from build123d import *

# Parameters (mm, degrees)
SKETCH1_R           = 50
SKETCH1_R_2         = 11.05
SKETCH1_R_3         = 1.55
BOSS_EXTRUDE1_DEPTH = 10
BOSS_EXTRUDE2_START = -2.9
SKETCH2_R           = 11.05
SKETCH2_R_2         = 4.05
BOSS_EXTRUDE2_DEPTH = 2.9


with BuildPart() as part:
    # Sketch1 → Boss-Extrude1 (new body)
    with BuildSketch(Plane.XY):
        Circle(SKETCH1_R)
        Circle(SKETCH1_R_2, mode=Mode.SUBTRACT)
        with Locations((40, 0)):
            Circle(SKETCH1_R_3, mode=Mode.SUBTRACT)
        with Locations((33.650141313, -21.625632698)):
            Circle(SKETCH1_R_3, mode=Mode.SUBTRACT)
        with Locations((16.61660052, -36.385279814)):
            Circle(SKETCH1_R_3, mode=Mode.SUBTRACT)
        with Locations((-5.692593531, -39.592857675)):
            Circle(SKETCH1_R_3, mode=Mode.SUBTRACT)
        with Locations((-26.194429358, -30.229982974)):
            Circle(SKETCH1_R_3, mode=Mode.SUBTRACT)
        with Locations((-38.379718945, -11.269302274)):
            Circle(SKETCH1_R_3, mode=Mode.SUBTRACT)
        with Locations((-38.379718945, 11.269302274)):
            Circle(SKETCH1_R_3, mode=Mode.SUBTRACT)
        with Locations((-26.194429358, 30.229982974)):
            Circle(SKETCH1_R_3, mode=Mode.SUBTRACT)
        with Locations((-5.692593531, 39.592857675)):
            Circle(SKETCH1_R_3, mode=Mode.SUBTRACT)
        with Locations((16.61660052, 36.385279814)):
            Circle(SKETCH1_R_3, mode=Mode.SUBTRACT)
        with Locations((33.650141313, 21.625632698)):
            Circle(SKETCH1_R_3, mode=Mode.SUBTRACT)
    extrude(amount=BOSS_EXTRUDE1_DEPTH)

    # Sketch2 → Boss-Extrude2 (add)
    with BuildSketch(Plane.XY.offset(10).offset(BOSS_EXTRUDE2_START)):
        Circle(SKETCH2_R)
        Circle(SKETCH2_R_2, mode=Mode.SUBTRACT)
    extrude(amount=BOSS_EXTRUDE2_DEPTH)


solid = part.part
Here's how the part is built. I have some questions about the finished solid (model axes, mm). A direction names the side the tool comes from. Coordinates: 2 decimals unless noted, no trailing zeros. Write each loop counter-clockwise with the first axis right and the second up, starting at its lowest first coordinate (ties: lowest second). Pieces come first, ordered by that corner, then holes.
1) Thinking about a two-plate mould opening in X: for faces 3 (the face through (-12, 1, 0)), 4 (the face through (34.365, 20.251, 4.93)), 5 (the face through (-5.89, 41.13, 4.93)), 6 (the face through (47.69, 15.02, 4.93)), which applies, +X half, -X half, draft (parallel to the pull), parting line (faces both ways), or undercut?
Filled in:
face 3: draft
face 4: undercut
face 5: undercut
face 6: parting line
2) If we section it at A-A (x = 40): List the corners of the cut face in (y, z) for me, plus the area to 3 significant figures.
Filled in:
outline: (-30, 0) - (-1.55, 0) - (-1.55, 10) - (-30, 10) - close; (1.55, 0) - (30, 0) - (30, 10) - (1.55, 10) - close
area: 569 mm2
3) If we section it at D-D (x = 0): List the corners of the cut face in (y, z) for me.
Filled in:
outline: (-50, 0) - (-11.05, 0) - (-11.05, 7.1) - (-4.05, 7.1) - (-4.05, 10) - (-50, 10) - close; (4.05, 7.1) - (11.05, 7.1) - (11.05, 0) - (50, 0) - (50, 10) - (4.05, 10) - close
4) I'm going to push flat-ended pins straight in: pin 1 (4 mm diameter, centred on y = -3.5, z = 2.5, fed in from -X); pin 2 (4 mm diameter, centred on x = -23.5, z = 7.5, fed in from -Y); pin 3 (3.5 mm diameter, centred on x = 16.62, y = 36.39, fed in from -Z); pin 4 (11 mm diameter, centred on x = 2, y = 0, fed in from -Z). Where does each tip first touch, or does it pass through?
Filled in:
pin 1: stops at x = -49.98
pin 2: stops at y = -45.14
pin 3: stops at z = 0
pin 4: stops at z = 7.1
5) Which directions (+Z, -Z, +X, -X, +Y, -Y) give clear straight access to the entire face, cutting with the end or side of a thin tool? Please do faces 1 (the face through (-1, -10, 10)), 2 (the face through (0, -5, 7.1)).
Filled in:
face 1: +Z, +X, -X, +Y, -Y
face 2: -Z
6) If we section it at B-B (y = 0): List the corners of the cut face in (x, z) for me.
Filled in:
outline: (-50, 0) - (-11.05, 0) - (-11.05, 7.1) - (-4.05, 7.1) - (-4.05, 10) - (-50, 10) - close; (4.05, 7.1) - (11.05, 7.1) - (11.05, 0) - (38.45, 0) - (38.45, 10) - (4.05, 10) - close; (41.55, 0) - (50, 0) - (50, 10) - (41.55, 10) - close
7) If I drill on line 1 (Y direction, x = -39.5, z = 5); line 2 (Y direction, x = 0, z = 3); line 3 (X direction, y = 39, z = 7.75), over which ranges is the centre line in solid material (lowest first)?
Filled in:
line 1: y = -30.66 to -12.34, -10.2 to 10.2, 12.34 to 30.66
line 2: y = -50 to -11.05, 11.05 to 50
line 3: x = -31.29 to -7.12, -4.26 to 31.29
8) If we section it at C-C (z = 3): Count the separate pieces of the cut face and the enclosed holes in it, plus the area to 3 significant figures.
Filled in:
separate pieces: 1
enclosed holes: 12
area: 7,390 mm2
